from build123d import *

# Parameters (mm, degrees)
ESQUISSE1_W             = 338
ESQUISSE1_H             = 335
BOSS_EXTRU_1_DEPTH      = 2
ESQUISSE2_W             = 318
ESQUISSE2_H             = 150
ESQUISSE2_W_2           = 90
ESQUISSE2_H_2           = 45
ENL_V_MAT_EXTRU_1_DEPTH = 238.952201082
D_GAGEMENT_M41_D        = 4.5
ESQUISSE5_W             = 3
ESQUISSE5_H             = 21.67
ENL_V_MAT_EXTRU_2_DEPTH = 238.952201082
ESQUISSE6_R             = 2.1
ENL_V_MAT_EXTRU_3_DEPTH = 238.952201082
ESQUISSE7_R             = 2.75
ENL_V_MAT_EXTRU_4_DEPTH = 238.952201082


with BuildPart() as part:
    # Esquisse1 → Boss.-Extru.1 (new body)
    with BuildSketch(Plane.XY):
        Rectangle(ESQUISSE1_W, ESQUISSE1_H)
    extrude(amount=BOSS_EXTRU_1_DEPTH)

    # Esquisse2 → Enlèv. mat.-Extru.1 (cut, through all)
    with BuildSketch(Plane.XY.offset(2)):
        with Locations((0, 92.5)):
            Rectangle(ESQUISSE2_W, ESQUISSE2_H)
        with Locations((124, -80)):
            Rectangle(ESQUISSE2_W_2, ESQUISSE2_H_2)
        with Locations((-124, -80)):
            Rectangle(ESQUISSE2_W_2, ESQUISSE2_H_2)
    extrude(amount=-ENL_V_MAT_EXTRU_1_DEPTH, mode=Mode.SUBTRACT)

    # Dégagement M41 (through all)
    with Locations(Plane.XY.offset(2)):
        with Locations((164, 129.17), (-164, 129.17)):
            Hole(D_GAGEMENT_M41_D / 2)

    # Esquisse5 → Enlèv. mat.-Extru.2 (cut, through all)
    with BuildSketch(Plane.XY.offset(2)):
        with Locations((157.5, 6.665)):
            Rectangle(ESQUISSE5_W, ESQUISSE5_H)
        with Locations((-157.5, 6.665)):
            Rectangle(ESQUISSE5_W, ESQUISSE5_H)
    extrude(amount=-ENL_V_MAT_EXTRU_2_DEPTH, mode=Mode.SUBTRACT)

    # Esquisse6 → Enlèv. mat.-Extru.3 (cut, through all)
    with BuildSketch(Plane.XY.offset(2)):
        with Locations((-164, 15.83)):
            Circle(ESQUISSE6_R)
        with Locations((-164, 145.83)):
            Circle(ESQUISSE6_R)
        with Locations(Location((164, 15.83, 0), (0, 0, 180))):
            Circle(ESQUISSE6_R)
        with Locations(Location((164, 145.83, 0), (0, 0, 180))):
            Circle(ESQUISSE6_R)
    extrude(amount=-ENL_V_MAT_EXTRU_3_DEPTH, mode=Mode.SUBTRACT)

    # Esquisse7 → Enlèv. mat.-Extru.4 (cut, through all)
    with BuildSketch(Plane.XY.offset(2)):
        with Locations((-120, -157.5)):
            Circle(ESQUISSE7_R)
        with Locations((-120, -14.17)):
            Circle(ESQUISSE7_R)
        with Locations(Location((120, -14.17, 0), (0, 0, 180))):
            Circle(ESQUISSE7_R)
        with Locations(Location((120, -157.5, 0), (0, 0, 180))):
            Circle(ESQUISSE7_R)
    extrude(amount=-ENL_V_MAT_EXTRU_4_DEPTH, mode=Mode.SUBTRACT)


solid = part.part
Check sheet for the modelled part. Datum: model origin and axes. Units: mm. Round coordinates to 2 decimals unless told otherwise and drop trailing zeros. Loops run counter-clockwise (first coordinate to the right, second up) from the corner with the lowest first, then second, coordinate; pieces in that order, holes last. Notation, with made-up numbers: M -24.5,65.5 L 19.5,65.5 A13 ccw 19.5,71.5 Z; hole C 61.25,57.25 d10. An arc over 180 degrees is marked long. One line per item, written item: value.
(1) Sectioned sample at C-C, the plane z = 1.6. Count the separate pieces of the cut face and the enclosed holes in it, then the cut area to 3 significant figures.
Computed values:
separate pieces: 1
enclosed holes: 10
area: 57,100 mm^2
(2) Sectioned sample at A-A, the plane x = -134.5. Record the cut outline in (y, z).
Computed values:
outline: M -167.5,0 L -102.5,0 L -102.5,2 L -167.5,2 Z; M -57.5,0 L 17.5,0 L 17.5,2 L -57.5,2 Z
(3) Sectioned sample at D-D, the plane x = -42. Record the cut outline in (y, z).
Computed values:
outline: M -167.5,0 L 17.5,0 L 17.5,2 L -167.5,2 Z
(4) Sectioned sample at B-B, the plane y = 54. Record the cut outline in (x, z).
Computed values:
outline: M -169,0 L -159,0 L -159,2 L -169,2 Z; M 159,0 L 169,0 L 169,2 L 159,2 Z
(5) Thickness scan on line 1 (Y direction, x = -120, z = 1.25); line 2 (X direction, y = 129.17, z = 1.1); line 3 (X direction, y = 3, z = 1.05). Record the ranges inside material, lowest first.
Computed values:
line 1: y = -167.5 to -160.25, -154.75 to -102.5, -57.5 to -16.92, -11.42 to 17.5
line 2: x = -169 to -166.25, -161.75 to -159, 159 to 161.75, 166.25 to 169
line 3: x = -169 to -159, -156 to 156, 159 to 169
(6) Depth check by flat-ended pin: pin 1 Ø1 at (y, z) = (-82, 0.5) entering from -X; pin 2 Ø1 at (x, z) = (12, 1) entering from +Y; pin 3 Ø0.6 at (x, z) = (158, 1) entering from +Y. Enter the tip coordinate at first touch or a pass-through.
Computed values:
pin 1: stops at x = -79
pin 2: stops at y = 17.5
pin 3: stops at y = -4.17
